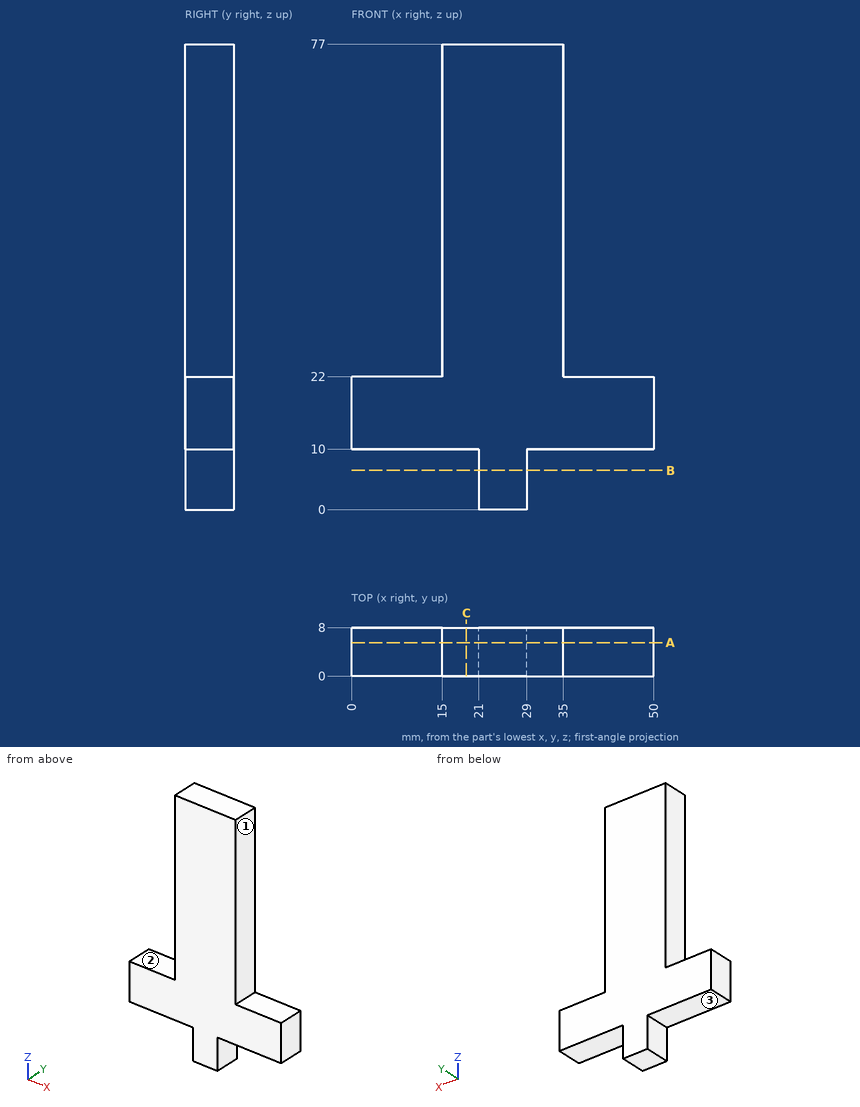
Can you work these out from the drawing? Everything is in mm from the part's minimum corner. A direction names the side the tool comes from. Coordinates: 2 decimals unless noted, no trailing zeros. Loops run counter-clockwise (first coordinate to the right, second up) from the corner with the lowest first, then second, coordinate; pieces in that order, holes last.
1. For the marked faces 1, 2 and 3, which set-ups out of +Z, -Z, +X, -X, +Y, -Y let a thin tool reach every point of the face, with its end or its side?
2. I need wall thicknesses on L1, parallel to Z at x = 48, y = 4.5; L2, parallel to X at y = 3, z = 34.5; L3, parallel to Z at x = 34.5, y = 4.5. Which ranges of each line are inside material? Lowest first, please.
3. Imagine slicing it at B-B, the plane z = 6.5. Please give me the cut outline in (x, y), and give its area (3 significant figures).
4. Imagine slicing it at A-A, the plane y = 5.5. Please give me the cut outline in (x, z), and give its area (3 significant figures).
5. Imagine slicing it at C-C, the plane x = 19. Please give me the cut outline in (y, z), and give its area (3 significant figures).
6. For P1, Ø4, axis at x = 43.5, y = 2.5, coming from the -Z side; P2, Ø4, axis at y = 5, z = 4.5, coming from the +X side; P3, Ø3, axis at y = 4.5, z = 52.5, coming from the -X side; P4, Ø3, axis at x = 23.5, z = 57, coming from the -Y side, each with a flat end and sliding along its axis, tell me the tip position at first contact or that it passes through.
Taken from the geometry:
1. face 1: +Z, +X, +Y, -Y
1. face 2: +Z, -X, +Y, -Y
1. face 3: -Z, -X, +Y, -Y
2. L1: z = 10 to 22
2. L2: x = 15 to 35
2. L3: z = 10 to 77
3. outline: (21, 0) - (29, 0) - (29, 8) - (21, 8) - close
3. area: 64.0 mm2
4. outline: (0, 10) - (21, 10) - (21, 0) - (29, 0) - (29, 10) - (50, 10) - (50, 22) - (35, 22) - (35, 77) - (15, 77) - (15, 22) - (0, 22) - close
4. area: 1,780 mm2
5. outline: (0, 10) - (8, 10) - (8, 77) - (0, 77) - close
5. area: 536 mm2
6. P1: stops at z = 10
6. P2: stops at x = 29
6. P3: stops at x = 15
6. P4: stops at y = 0
